Design review of the part built by this model. Coordinates are the model's own, in mm. A direction names the side the tool comes from. Round coordinates to 2 decimals unless told otherwise and drop trailing zeros. Loops run counter-clockwise (first coordinate to the right, second up) from the corner with the lowest first, then second, coordinate; pieces in that order, holes last. Notation, with made-up numbers: M 88,17 L 131,17 A12 cw 131,37 Z; hole C 45,-29.75 d4. An arc over 180 degrees is marked long. Use a Markdown table: item, result.
from build123d import *

# Parameters (mm, degrees)
BOSS_EXTRUDE1_DEPTH  = 30
SHELL1_T             = -7
SKETCH2_R            = 15
CUT_EXTRUDE1_DEPTH   = 20
SKETCH3_R            = 2.805999004
CUT_EXTRUDE2_DEPTH   = 20
LPATTERN1_COUNT      = 2
LPATTERN1_PITCH      = 47
LPATTERN1_COUNT_DIR2 = 2
LPATTERN1_PITCH_DIR2 = 47
SKETCH4_W            = 37.798746628
SKETCH4_H            = 38.365375912
CUT_EXTRUDE3_DEPTH   = 4
SKETCH5_R            = 9.689386482
CUT_EXTRUDE4_DEPTH   = 10
SKETCH6_R            = 2.109382838
CUT_EXTRUDE5_DEPTH   = 10
LPATTERN2_COUNT      = 2
LPATTERN2_PITCH      = 25
LPATTERN2_COUNT_DIR2 = 2
LPATTERN2_PITCH_DIR2 = 25
SKETCH7_R            = 3.099977118
CUT_EXTRUDE6_DEPTH   = 10
LPATTERN3_COUNT      = 3
LPATTERN3_PITCH      = 60
SKETCH8_R            = 3.106688242
CUT_EXTRUDE7_DEPTH   = 10
LPATTERN4_COUNT      = 3
LPATTERN4_PITCH      = 40


with BuildPart() as part:
    # Sketch1 → Boss-Extrude1 (new body)
    with BuildSketch(Plane.XY):
        with BuildLine():
            Line((-48.579903717, 70.777906396), (-98.579903717, 20.777906396))
            Line((-98.579903717, 20.777906396), (-98.579903717, -49.222093604))
            Line((-98.579903717, -49.222093604), (81.420096283, -49.222093604))
            Line((81.420096283, -49.222093604), (81.420096283, 69.777906396))
            ThreePointArc((81.420096283, 69.777906396), (81.127203064, 70.485013177), (80.420096283, 70.777906396))
            Line((80.420096283, 70.777906396), (-48.579903717, 70.777906396))
        make_face()
    extrude(amount=BOSS_EXTRUDE1_DEPTH)

    # Shell1
    shell1_openings = [part.faces().sort_by_distance(p)[0] for p in [
        (-4.076298463, 8.11549528, 30),
    ]]
    offset(amount=SHELL1_T, openings=shell1_openings, kind=Kind.INTERSECTION)

    # Sketch2 → Cut-Extrude1 (cut)
    with BuildSketch(Plane.XY.offset(7)):
        with Locations((-58.579903717, -9.222093604)):
            Circle(SKETCH2_R)
    extrude(amount=-CUT_EXTRUDE1_DEPTH, mode=Mode.SUBTRACT)

    # Sketch3 → Cut-Extrude2 (cut)
    with BuildSketch(Plane.XY.offset(7)):
        with Locations((-82.079903717, 14.277906396)):
            Circle(SKETCH3_R)
    cut_extrude2 = extrude(amount=-CUT_EXTRUDE2_DEPTH, mode=Mode.SUBTRACT)

    # LPattern1: Cut-Extrude2 2 × 2
    with Locations(*[(i * LPATTERN1_PITCH, -j * LPATTERN1_PITCH_DIR2, 0) for i in range(LPATTERN1_COUNT) for j in range(LPATTERN1_COUNT_DIR2) if (i, j) != (0, 0)]):
        add(cut_extrude2, mode=Mode.SUBTRACT)

    # Sketch4 → Cut-Extrude3 (cut)
    with BuildSketch(Plane.XY.offset(7)):
        with Locations((11.520722969, 29.59521844)):
            Rectangle(SKETCH4_W, SKETCH4_H)
    extrude(amount=-CUT_EXTRUDE3_DEPTH, mode=Mode.SUBTRACT)

    # Sketch5 → Cut-Extrude4 (cut)
    with BuildSketch(Plane(origin=(0, 0, 5), x_dir=(-1, 0, 0), z_dir=(0, 0, -1))):
        with Locations(Location((-1.55943854, 29.087809619, 0), (0, 0, 337.288675779))):
            Circle(SKETCH5_R)
    extrude(amount=CUT_EXTRUDE4_DEPTH, mode=Mode.SUBTRACT)

    # Sketch6 → Cut-Extrude5 (cut)
    with BuildSketch(Plane(origin=(0, 0, 5), x_dir=(-1, 0, 0), z_dir=(0, 0, -1))):
        with Locations(Location((-14.05943854, 41.587809619, 0), (0, 0, 180))):
            Circle(SKETCH6_R)
    cut_extrude5 = extrude(amount=CUT_EXTRUDE5_DEPTH, mode=Mode.SUBTRACT)

    # LPattern2: Cut-Extrude5 2 × 2
    with Locations(*[(-i * LPATTERN2_PITCH, -j * LPATTERN2_PITCH_DIR2, 0) for i in range(LPATTERN2_COUNT) for j in range(LPATTERN2_COUNT_DIR2) if (i, j) != (0, 0)]):
        add(cut_extrude5, mode=Mode.SUBTRACT)

    # Sketch7 → Cut-Extrude6 (cut)
    with BuildSketch(Plane.XZ.offset(49.222093604)):
        with Locations(Location((-68.579903717, 15, 0), (0, 0, 270))):
            Circle(SKETCH7_R)
    cut_extrude6 = extrude(amount=-CUT_EXTRUDE6_DEPTH, mode=Mode.SUBTRACT)

    # LPattern3: Cut-Extrude6 ×3
    with Locations(*[(i * LPATTERN3_PITCH, 0, 0) for i in range(1, LPATTERN3_COUNT)]):
        add(cut_extrude6, mode=Mode.SUBTRACT)

    # Sketch8 → Cut-Extrude7 (cut)
    with BuildSketch(Plane(origin=(81.420096283, 0, 0), x_dir=(0, 0, -1), z_dir=(1, 0, 0))):
        with Locations(Location((-15.098987318, -32.974488262, 0), (0, 0, 90))):
            Circle(SKETCH8_R)
    cut_extrude7 = extrude(amount=-CUT_EXTRUDE7_DEPTH, mode=Mode.SUBTRACT)

    # LPattern4: Cut-Extrude7 ×3
    with Locations(*[(0, i * LPATTERN4_PITCH, 0) for i in range(1, LPATTERN4_COUNT)]):
        add(cut_extrude7, mode=Mode.SUBTRACT)


solid = part.part
1. Wall thickness on line 1 along X through (y, z) = (-43.75, 15); line 2 along X through (y, z) = (-17, 24); line 3 along Y through (x, z) = (32.5, 16.25): over which ranges is each line inside the solid? List them lowest first. Write a range as from..to.
Check values:
| item | result |
|---|---|
| line 1 | x = -98.58..-71.68, -65.48..-11.68, -5.48..48.32, 54.52..81.42 |
| line 2 | x = -98.58..-91.58, 74.42..81.42 |
| line 3 | y = -49.22..-42.22, 63.78..70.78 |
2. Machinability: for faces 5 (the face through (11, 48.778, 5)), 6 (the face through (-9.807, 39.809, 2.535)), 7 (the face through (-73.23, 46.13, 14.79)), which of the approach directions +Z, -Z, +X, -X, +Y, -Y give a long, thin tool a straight path to every point of the face, cutting with its end or side? Answer none if there is none.
Check values:
| item | result |
|---|---|
| face 5 | +Z |
| face 6 | -Z |
| face 7 | +Z, -Z, -X, +Y |
3. Take a section at A-A on y = 30.5. Give the boundary of the cut face in (x, z).
Check values:
| item | result |
|---|---|
| outline | M -88.86,0 L -8.03,0 L -8.03,5 L -7.38,5 L -7.38,7 L -78.96,7 L -78.96,30 L -88.86,30 Z; M 11.15,0 L 81.42,0 L 81.42,30 L 74.42,30 L 74.42,7 L 30.42,7 L 30.42,3 L 11.15,3 Z |
4. The part is to be moulded in two halves that separate along Z. For faces 1 (the face through (15, 30, 3)), 2 (the face through (-11, 42, 5)), 3 (the face through (-84.307, 12.57, 3.549)), 4 (the face through (-71.33, -45.77, 13.57)), say which applies: pulls with the +Z half, pulls with the -Z half, needs draft (parallel to the pull), parting line crosses it, or undercut.
Check values:
| item | result |
|---|---|
| face 1 | pulls with the +Z half |
| face 2 | pulls with the -Z half |
| face 3 | needs draft |
| face 4 | undercut |
5. Take a section at B-B on x = 27. Give the boundary of the cut face in (y, z), and give its area (3 significant figures).
Check values:
| item | result |
|---|---|
| outline | M -49.22,0 L 70.78,0 L 70.78,30 L 63.78,30 L 63.78,7 L 48.78,7 L 48.78,3 L 10.41,3 L 10.41,7 L -42.22,7 L -42.22,30 L -49.22,30 Z |
| area | 1,010 mm² |
6. Take a section at C-C on z = 27.5. Give the boundary of the cut face in (x, y).
Check values:
| item | result |
|---|---|
| outline | M -98.58,-49.22 L 81.42,-49.22 L 81.42,69.78 A1 ccw 80.42,70.78 L -48.58,70.78 L -98.58,20.78 Z; hole M -91.58,-42.22 L 74.42,-42.22 L 74.42,63.78 L -45.68,63.78 L -91.58,17.88 Z |
7. Insertion check: pin 1 (2 mm diameter, centred on x = -15.5, y = 18.5, fed in from -Z); pin 2 (1.5 mm diameter, centred on x = 14.5, y = 3, fed in from +Z); pin 3 (3.5 mm diameter, centred on y = 47.03, z = 15.1, fed in from +X); pin 4 (5 mm diameter, centred on x = -68.58, z = 15, fed in from -Y). Each pin has a flat end and moves straight along its axis. Give the tip position at first contact, or say it passes through.
Check values:
| item | result |
|---|---|
| pin 1 | stops at z = 0 |
| pin 2 | stops at z = 7 |
| pin 3 | stops at x = -60.68 |
| pin 4 | stops at y = 38.38 |
8. Take a section at D-D on y = -27. Give the boundary of the cut face in (x, z), and give its area (3 significant figures).
Check values:
| item | result |
|---|---|
| outline | M -98.58,0 L 81.42,0 L 81.42,30 L 74.42,30 L 74.42,7 L -91.58,7 L -91.58,30 L -98.58,30 Z |
| area | 1,580 mm² |
